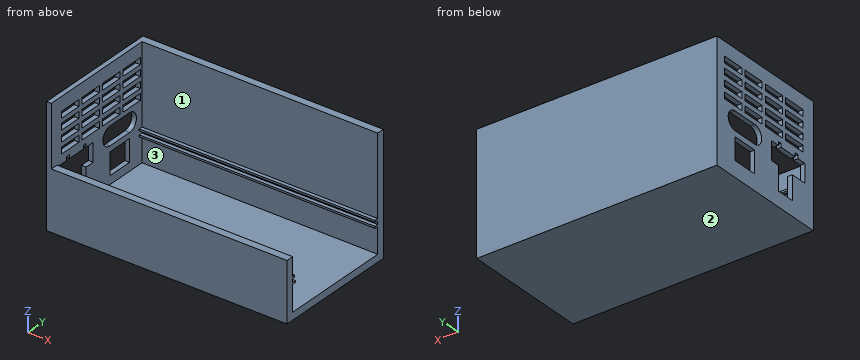
```python
from build123d import *

# Parameters (mm, degrees)
F1_DEPTH = 130
F2_W     = 69
F2_H     = 65
F2_W_2   = 14
F2_H_2   = 12
F2_W_3   = 12.5
F2_H_3   = 3.5
F3_DEPTH = 2.5


with BuildPart() as f1:
    # F0 (on Right) → F1 (new body)
    with BuildSketch(Plane.YZ):
        Polygon((0, 32), (0, 0), (69, 0), (69, 65), (65, 65), (65, 22), (63, 22), (63, 21), (65, 21), (65, 19), (63, 19), (63, 18), (65, 18), (65, 4), (4, 4), (4, 18), (6, 18), (6, 19), (4, 19), (4, 21), (5.5, 21), (5.5, 22), (4, 22), (4, 32), align=None)
    extrude(amount=F1_DEPTH)

    # F2 (on face) → F3 (join)
    with BuildSketch(Plane(origin=(0, 0, 0), x_dir=(0, -1, 0), z_dir=(-1, 0, 0))):
        with Locations((-34.5, 32.5)):
            Rectangle(F2_W, F2_H)
        with Locations((-49, 14.5)):
            Rectangle(F2_W_2, F2_H_2, mode=Mode.SUBTRACT)
        with BuildLine():
            Line((-42, 23.5), (-56, 23.5))
            ThreePointArc((-56, 23.5), (-61, 28.5), (-56, 33.5))
            Line((-56, 33.5), (-42, 33.5))
            ThreePointArc((-42, 33.5), (-37, 28.5), (-42, 23.5))
        make_face(mode=Mode.SUBTRACT)
        Polygon((-11, 31), (-6, 31), (-6, 21), (-15, 21), (-15, 8), (-25, 8), (-25, 21), (-30, 21), (-30, 31), (-25, 31), (-25, 33), (-23, 33), (-23, 31), (-13, 31), (-13, 33), (-11, 33), align=None, mode=Mode.SUBTRACT)
        with Locations((-57.5, 37.75)):
            Rectangle(F2_W_3, F2_H_3, mode=Mode.SUBTRACT)
        with Locations((-57.5, 43.75)):
            Rectangle(F2_W_3, F2_H_3, mode=Mode.SUBTRACT)
        with Locations((-42.833333, 37.75)):
            Rectangle(F2_W_3, F2_H_3, mode=Mode.SUBTRACT)
        with Locations((-42.833333, 43.75)):
            Rectangle(F2_W_3, F2_H_3, mode=Mode.SUBTRACT)
        with Locations((-57.5, 49.75)):
            Rectangle(F2_W_3, F2_H_3, mode=Mode.SUBTRACT)
        with Locations((-57.5, 55.75)):
            Rectangle(F2_W_3, F2_H_3, mode=Mode.SUBTRACT)
        with Locations((-42.833333, 49.75)):
            Rectangle(F2_W_3, F2_H_3, mode=Mode.SUBTRACT)
        with Locations((-42.833333, 55.75)):
            Rectangle(F2_W_3, F2_H_3, mode=Mode.SUBTRACT)
        with Locations((-28.166667, 37.75)):
            Rectangle(F2_W_3, F2_H_3, mode=Mode.SUBTRACT)
        with Locations((-28.166667, 43.75)):
            Rectangle(F2_W_3, F2_H_3, mode=Mode.SUBTRACT)
        with Locations((-13.5, 37.75)):
            Rectangle(F2_W_3, F2_H_3, mode=Mode.SUBTRACT)
        with Locations((-13.5, 43.75)):
            Rectangle(F2_W_3, F2_H_3, mode=Mode.SUBTRACT)
        with Locations((-28.166667, 49.75)):
            Rectangle(F2_W_3, F2_H_3, mode=Mode.SUBTRACT)
        with Locations((-28.166667, 55.75)):
            Rectangle(F2_W_3, F2_H_3, mode=Mode.SUBTRACT)
        with Locations((-13.5, 49.75)):
            Rectangle(F2_W_3, F2_H_3, mode=Mode.SUBTRACT)
        with Locations((-13.5, 55.75)):
            Rectangle(F2_W_3, F2_H_3, mode=Mode.SUBTRACT)
    extrude(amount=-F3_DEPTH)


solid = f1.part
```
Work out the finished part from the listing and answer in its coordinate system (mm). Face numbers are marked on the shaded views. Round coordinates to 2 decimals unless told otherwise and drop trailing zeros. Loops run counter-clockwise (first coordinate to the right, second up) from the corner with the lowest first, then second, coordinate; pieces in that order, holes last. Notation, with made-up numbers: (34, 67.5) -> (48, 67.5) arc R17 ccw to (48, 82.5) -> close; hole circle Ø2 at (14, 11.5). An arc over 180 degrees is marked (long way). Write each question's results on one line, items separated by ' | '. Start each with the question number.
1. For a pull along Z with two mould halves and no side action, classify the marked faces 1, 2 and 3 as +Z half, -Z half, draft (parallel to the pull), parting line (faces both ways), or undercut.
2. Given pin 1 Ø3 at (x, y) = (1.5, 9) entering from -Z; pin 2 Ø4 at (y, z) = (44, 23) entering from +X; pin 3 Ø0.6 at (x, y) = (75.5, 64) entering from +Z; pin 4 Ø10 at (x, z) = (113, 56.5) entering from -Y, each flat-ended and moving along its own axis, determine where each tip first touches the part or whether it passes through.
3. Find the intervals of material crossed by probe 1 along Y at (x, z) = (101, 15); probe 2 along Y at (x, z) = (121.5, 59.5); probe 3 along X at (y, z) = (47, 47), in increasing order. Write a range as from..to.
4. Section B-B (x = 106) is taken. Determine the outline of the cut face in (y, z).
5. Section A-A (z = 28.5) is taken. Determine the outline of the cut face in (x, y), plus the area to 3 significant figures.
Evaluation:
1) face 1: draft | face 2: -Z half | face 3: undercut
2) pin 1: stops at z = 0 | pin 2: stops at x = 2.5 | pin 3: stops at z = 22 | pin 4: stops at y = 65
3) probe 1: y = 0..4, 65..69 | probe 2: y = 65..69 | probe 3: x = 0..2.5
4) outline: (0, 0) -> (69, 0) -> (69, 65) -> (65, 65) -> (65, 22) -> (63, 22) -> (63, 21) -> (65, 21) -> (65, 19) -> (63, 19) -> (63, 18) -> (65, 18) -> (65, 4) -> (4, 4) -> (4, 18) -> (6, 18) -> (6, 19) -> (4, 19) -> (4, 21) -> (5.5, 21) -> (5.5, 22) -> (4, 22) -> (4, 32) -> (0, 32) -> close
5) outline: (0, 0) -> (130, 0) -> (130, 4) -> (2.5, 4) -> (2.5, 6) -> (0, 6) -> close; (0, 30) -> (2.5, 30) -> (2.5, 37) -> (0, 37) -> close; (0, 61) -> (2.5, 61) -> (2.5, 65) -> (130, 65) -> (130, 69) -> (0, 69) -> close | area: 1,070 mm2
